```python
from build123d import *

# Parameters (mm, degrees)
F0_W     = 38.1
F0_H     = 38.1
F1_DEPTH = 19.05
F2_R     = 10.862453
F3_DEPTH = 25.4


with BuildPart() as f1:
    # F0 (on Front) → F1 (new body, symmetric)
    with BuildSketch(Plane.XZ):
        with Locations((-19.05, 19.05)):
            Rectangle(F0_W, F0_H)
    extrude(amount=F1_DEPTH, both=True)

    # F2 (on face) → F3 (join)
    with BuildSketch(Plane.YZ):
        with Locations((0, 18.468129)):
            Circle(F2_R)
    extrude(amount=F3_DEPTH)


solid = f1.part
```
Here's how the part is built. I have some questions about the finished solid (model axes, mm). A direction names the side the tool comes from. Round coordinates to 2 decimals unless told otherwise and drop trailing zeros. Loops run counter-clockwise (first coordinate to the right, second up) from the corner with the lowest first, then second, coordinate; pieces in that order, holes last.
1. Will these pins go through, and if not, where does the flat tip stop? pin 1 (3 mm diameter, centred on x = 12.5, z = 11, fed in from +Y); pin 2 (10 mm diameter, centred on y = 15, z = 27, fed in from +X).
Answers:
pin 1: stops at y = 9.08
pin 2: stops at x = 0
2. Suppose I cut it at C-C, the plane x = 6. Please give me the cut outline in (y, z), and give its area (3 significant figures).
Answers:
outline: circle Ø21.72 at (0, 18.47)
area: 371 mm2
3. Suppose I cut it at B-B, the plane z = 24. Please give me the cut outline in (x, y).
Answers:
outline: (-38.1, -19.05) - (0, -19.05) - (0, -9.35) - (25.4, -9.35) - (25.4, 9.35) - (0, 9.35) - (0, 19.05) - (-38.1, 19.05) - close
4. Suppose I cut it at A-A, the plane y = 0. Please give me the cut outline in (x, z).
Answers:
outline: (-38.1, 0) - (0, 0) - (0, 7.61) - (25.4, 7.61) - (25.4, 29.33) - (0, 29.33) - (0, 38.1) - (-38.1, 38.1) - close
5. Suppose I cut it at D-D, the plane z = 5.5. Please give me the cut outline in (x, y).
Answers:
outline: (-38.1, -19.05) - (0, -19.05) - (0, 19.05) - (-38.1, 19.05) - close
6. For faces 1 (the face through (25.4, 0, 19)), 2 (the face through (12.522, -2.355, 7.864)), which set-ups out of +Z, -Z, +X, -X, +Y, -Y let a thin tool reach every point of the face, with its end or its side?
Answers:
face 1: +Z, -Z, +X, +Y, -Y
face 2: +X
7. If I drill on probe 1 along X at (y, z) = (11.5, 23); probe 2 along Z at (x, y) = (21, 9.5); probe 3 along Y at (x, z) = (22, 11.5), over which ranges is the centre line in solid material (lowest first)?
Answers:
probe 1: x = -38.1 to 0
probe 2: z = 13.2 to 23.74
probe 3: y = -8.33 to 8.33
